The model under review builds one solid part; all positions refer to its coordinate system, in mm. A direction names the side the tool comes from. Give positions to 0.01 mm unless a question says otherwise; leave off trailing zeros. Write each loop counter-clockwise with the first axis right and the second up, starting at its lowest first coordinate (ties: lowest second). Pieces come first, ordered by that corner, then holes. Notation, with made-up numbers: (-29.75, 61.25) - (-2.75, 61.25) arc R20 cw to (-2.75, 65.25) - close; hole circle Ø2 at (12, 50). An arc over 180 degrees is marked (long way). One line per question, with ' | ' between items. Start each with the question number.
```python
from build123d import *

# Parameters (mm, degrees)
HEX_2_DEPTH = 2.3876


# Read off the part's stored shape, not the designer's step: ThreadSchematic
with BuildPart() as part:
    # ThreadSchematic outline → ThreadSchematic (revolve)
    with BuildSketch(Plane.YX):
        with BuildLine():
            Line((0, 39.7002), (0, 0))
            Line((0, 0), (3.9751, 0))
            Line((3.9751, 0), (4.7625, 0.7874))
            Line((4.7625, 0.7874), (4.7625, 4.7752))
            Line((4.7625, 4.7752), (3.1115, 4.7752))
            ThreePointArc((3.1115, 4.7752), (2.94985539, 4.84215539), (2.8829, 5.0038))
            Line((2.8829, 5.0038), (2.8829, 6.8707))
            Line((2.8829, 6.8707), (3.1496, 7.1374))
            Line((3.1496, 7.1374), (3.1496, 30.1752))
            Line((3.1496, 30.1752), (2.2733, 30.1752))
            ThreePointArc((2.2733, 30.1752), (1.860208218, 30.346308218), (1.6891, 30.7594))
            Line((1.6891, 30.7594), (1.6891, 32.2834))
            Line((1.6891, 32.2834), (2.413, 33.0073))
            Line((2.413, 33.0073), (2.413, 39.07028))
            Line((2.413, 39.07028), (1.78308, 39.7002))
            Line((1.78308, 39.7002), (0, 39.7002))
        make_face()
    revolve(axis=Axis((0, 0, 0), (1, 0, 0)))

    # Sketch2 → PreBroach (revolve, cut)
    with BuildSketch(Plane.XY, mode=Mode.PRIVATE) as prebroach_sk:
        Polygon((0, 1.5875), (2.3876, 1.5875), (3.304143552, 0), (0, 0), align=None)
    revolve(prebroach_sk.sketch.rotate(Axis((0, 0, 0), (1, 0, 0)), 90), axis=Axis((0, 0, 0), (1, 0, 0)), mode=Mode.SUBTRACT)

    # Sketch3 → Hex 2 (cut)
    with BuildSketch(Plane.ZY):
        Polygon((-1.5875, -0.916543552), (-1.5875, 0.916543552), (0, 1.833087105), (1.5875, 0.916543552), (1.5875, -0.916543552), (0, -1.833087105), align=None)
    extrude(amount=-HEX_2_DEPTH, mode=Mode.SUBTRACT)


solid = part.part
```
Item 1: Clearance check with flat-ended pins moving along their axes: P1, Ø1, axis at y = 2, z = 2.5, coming from the +X side; P2, Ø1, axis at x = 19.5, y = 3, coming from the +Z side; P3, Ø3, axis at x = 8.5, z = 1.5, coming from the -Y side. State where each tip first meets the part, or that it passes through.
Item 2: For probe 1 along X at (y, z) = (-3.25, -2.25); probe 2 along Z at (x, y) = (11.5, -0.5); probe 3 along X at (y, z) = (2.25, 1.5), list the stretches that pass through material, from the lowest coordinate up.
Item 3: The part is to be moulded in two halves that separate along X. For faces 5 (the cylindrical face through (31.53, -1.34, -1.03)), 6 (the flat face through (1.18, -1.37, 0.8)), 7 (the flat face through (0, 0, -2)), 8 (the flat face through (39.7, 0, 0)), say which applies: +X half, -X half, draft (parallel to the pull), parting line (faces both ways), or undercut.
Item 4: Machinability: for faces 1 (the cylindrical face through (2.81, -3.78, -2.9)), 2 (the cylindrical face through (5.95, -2.88, 0.13)), 3 (the flat face through (1.177, -1.381, -0.783)), 4 (the cylindrical face through (36.081, -1.915, -1.468)), which of the approach directions +Z, -Z, +X, -X, +Y, -Y give a long, thin tool a straight path to every point of the face, cutting with its end or side? Answer none if there is none.
Item 5: Take a section at A-A (x = 29). Give the boundary of the cut face in (y, z).
Item 6: Take a section at B-B (x = 6). Give the boundary of the cut face in (y, z).
Check sheet entries:
1) P1: stops at x = 30.18 | P2: stops at z = 1.92 | P3: stops at y = -3.15
2) probe 1: x = 0 to 4.78 | probe 2: z = -3.11 to 3.11 | probe 3: x = 0 to 30.18
3) face 5: undercut | face 6: draft | face 7: -X half | face 8: +X half
4) face 1: +X, -X | face 2: none | face 3: -X | face 4: +X
5) outline: circle Ø6.3 at (0, 0)
6) outline: circle Ø5.77 at (0, 0)
